```python
from build123d import *

# Parameters (mm, degrees)
SKETCH_1_W          = 215
SKETCH_1_H          = 100
EXTRUDE_1_DEPTH     = 1.5
SKETCH_2_W          = 155
SKETCH_2_H          = 140
CUT_EXTRUDE_1_DEPTH = 21.5
FILLET_1_R          = 30
SKETCH_3_R          = 1.525
CUT_EXTRUDE_2_DEPTH = 10
SKETCH_4_R          = 1.525
CUT_EXTRUDE_3_DEPTH = 10


with BuildPart() as part:
    # 草图1 → 凸台-拉伸1 (new body, symmetric)
    with BuildSketch(Plane.XY):
        Rectangle(SKETCH_1_W, SKETCH_1_H)
    extrude(amount=EXTRUDE_1_DEPTH, both=True)

    # 草图2 → 切除-拉伸1 (cut, symmetric)
    with BuildSketch(Plane.XY.offset(1.5)):
        with Locations((0, 50)):
            Rectangle(SKETCH_2_W, SKETCH_2_H)
    extrude(amount=CUT_EXTRUDE_1_DEPTH, both=True, mode=Mode.SUBTRACT)

    # 圆角1
    fillet_1_edges = [part.edges().sort_by_distance(p)[0] for p in [
        (77.5, -20, 0),
        (-77.5, -20, 0),
    ]]
    fillet(fillet_1_edges, radius=FILLET_1_R)

    # 草图3 → 切除-拉伸2 (cut)
    with BuildSketch(Plane(origin=(0, 0, -1.5), x_dir=(-1, 0, 0), z_dir=(0, 0, -1))):
        with Locations((-5, -44)):
            Circle(SKETCH_3_R)
        with Locations((15, -44)):
            Circle(SKETCH_3_R)
    extrude(amount=-CUT_EXTRUDE_2_DEPTH, mode=Mode.SUBTRACT)

    # 草图4 → 切除-拉伸3 (cut)
    with BuildSketch(Plane.XY.offset(1.5)):
        with Locations((-104.5, 16.5)):
            Circle(SKETCH_4_R)
        with Locations((-104.5, -3.5)):
            Circle(SKETCH_4_R)
    cut_extrude_3 = extrude(amount=-CUT_EXTRUDE_3_DEPTH, mode=Mode.SUBTRACT)

    # 镜向1: 切除-拉伸3 across plane
    add(cut_extrude_3.mirror(Plane(origin=(0, 0, 0), x_dir=(0, 0, 1), z_dir=(1, 0, 0))), mode=Mode.SUBTRACT)


solid = part.part
```
CAD build for the part. Positions are in the model's coordinates, mm. Round coordinates to 2 decimals unless told otherwise and drop trailing zeros. Loops run counter-clockwise (first coordinate to the right, second up) from the corner with the lowest first, then second, coordinate; pieces in that order, holes last. Notation, with made-up numbers: M 58,-7 L 111,-7 A24 cw 111,4 Z; hole C -29.5,52 d5. An arc over 180 degrees is marked long. Return JSON: item names as keys, results as strings. Group by question number.
(1) Saw through at C-C, the plane y = 6. List the corners of the cut face in (x, z).
(2) Drop flat-ended pins along their axis: P1, Ø1, axis at x = -16, z = 0.5, coming from the +Y side; P2, Ø2.5, axis at x = 104.5, y = -3.5, coming from the -Z side. Give the stop position or say it passes through.
(3) Saw through at B-B, the plane z = -0.8. List the corners of the cut face in (x, y) (3 decimals), and give its area (3 significant figures).
(4) Saw through at A-A, the plane y = 42. List the corners of the cut face in (x, z), and give its area (3 significant figures).
(5) Mould opens along X. For faces 1 (the flat face through (-2, -22, -1.5)), 2 (the cylindrical face through (68.479, -11.445, 0.021)), 3 (the cylindrical face through (-68.945, -10.979, 0.021)) say: +X half, -X half, draft (parallel to the pull), parting line (faces both ways), or undercut.
(6) Saw through at D-D, the plane x = -2.5. List the corners of the cut face in (y, z).
(7) Wall check: probe 1 along Y at (x, z) = (-104.5, -0.2) (3 decimals); probe 2 along Y at (x, z) = (-15, 0.45) (3 decimals); probe 3 along X at (y, z) = (36.5, 1.25). Give the ranges that are in metal, low to high. Write a range as [from, to].
Answer list:
{
 "1": {"outline": "M -107.5,-1.5 L -77.23,-1.5 L -77.23,1.5 L -107.5,1.5 Z; M 77.23,-1.5 L 107.5,-1.5 L 107.5,1.5 L 77.23,1.5 Z"},
 "2": {"P1": "y = -20", "P2": "through"},
 "3": {"outline": "M -107.5,-50 L 107.5,-50 L 107.5,50 L 77.5,50 L 77.5,10 A30 cw 47.5,-20 L -47.5,-20 A30 cw -77.5,10 L -77.5,50 L -107.5,50 Z; hole C -104.5,-3.5 d3.05; hole C -104.5,16.5 d3.05; hole C -15,-44 d3.05; hole C 5,-44 d3.05; hole C 104.5,-3.5 d3.05; hole C 104.5,16.5 d3.05", "area": "11,000 mm2"},
 "4": {"outline": "M -107.5,-1.5 L -77.5,-1.5 L -77.5,1.5 L -107.5,1.5 Z; M 77.5,-1.5 L 107.5,-1.5 L 107.5,1.5 L 77.5,1.5 Z", "area": "180 mm2"},
 "5": {"face 1": "draft", "face 2": "undercut", "face 3": "undercut"},
 "6": {"outline": "M -50,-1.5 L -20,-1.5 L -20,1.5 L -50,1.5 Z"},
 "7": {"probe 1": "[-50, -5.025], [-1.975, 14.975], [18.025, 50]", "probe 2": "[-50, -45.525], [-42.475, -20]", "probe 3": "[-107.5, -77.5], [77.5, 107.5]"}
}
